```python
from build123d import *

# Parameters (mm, degrees)
SALIENTE_EXTRUIR1_DEPTH = 2.5
SALIENTE_EXTRUIR2_DEPTH = 2.5
CROQUIS3_R              = 2.25
CROQUIS3_W              = 4
CROQUIS3_H              = 100.57
CORTAR_EXTRUIR1_DEPTH   = 10
CORTAR_EXTRUIR3_DEPTH   = 82
CORTAR_EXTRUIR4_DEPTH   = 90


with BuildPart() as part:
    # Croquis1 → Saliente-Extruir1 (new body)
    with BuildSketch(Plane(origin=(0, 0, 0), x_dir=(0, 0, -1), z_dir=(1, 0, 0))):
        Polygon((-49.88, -57.285), (49.88, -57.285), (81.7, -24.565), (81.7, 25.235), (49.65, 57.285), (-49.95, 57.285), (-81.7, 24.905), (-81.7, -24.565), align=None)
    extrude(amount=SALIENTE_EXTRUIR1_DEPTH)

    # Croquis2 → Saliente-Extruir2 (add)
    with BuildSketch(Plane(origin=(2.5, 0, 0), x_dir=(0, 0, -1), z_dir=(1, 0, 0))):
        Polygon((81.7, 25.235), (49.65, 57.285), (60.256601718, 67.891601718), (92.306601718, 35.841601718), align=None)
        Polygon((-81.7, 24.905), (-49.95, 57.285), (-60.660282007, 67.786897892), (-92.410282007, 35.406897892), align=None)
        Polygon((-81.7, -24.565), (-49.88, -57.285), (-60.633463585, -67.742677606), (-92.453463585, -35.022677606), align=None)
        Polygon((49.88, -57.285), (81.7, -24.565), (92.453463585, -35.022677606), (60.633463585, -67.742677606), align=None)
    extrude(amount=-SALIENTE_EXTRUIR2_DEPTH)

    # Croquis3 → Cortar-Extruir1 (cut)
    with BuildSketch(Plane(origin=(2.5, 0, 0), x_dir=(0, 0, -1), z_dir=(1, 0, 0))):
        with Locations((-76.540373615, 33.850995118)):
            Circle(CROQUIS3_R)
        with Locations((-59.042204467, 51.550828198)):
            Circle(CROQUIS3_R)
        with Locations((76.301473252, 34.051102275)):
            Circle(CROQUIS3_R)
        with Locations((58.757017396, 51.705056035)):
            Circle(CROQUIS3_R)
        with Locations((76.369576687, -33.391936282)):
            Circle(CROQUIS3_R)
        with Locations((58.860810215, -51.081286502)):
            Circle(CROQUIS3_R)
        with Locations((-58.938482889, -51.164964143)):
            Circle(CROQUIS3_R)
        with Locations((-76.472362613, -33.500506143)):
            Circle(CROQUIS3_R)
        with BuildLine():
            Line((-8.35, 0), (-8.35, -10.698407243))
            Line((-8.35, -10.698407243), (8.347094832, -10.698407243))
            Line((8.347094832, -10.698407243), (8.321717757, -0.686668462))
            ThreePointArc((8.321717757, -0.686668462), (0.343625327, 8.342926443), (-8.35, 0))
        make_face()
        Polygon((23.469483411, 50.346823407), (23.732824148, -50.222831816), (27.732810435, -50.212357888), (27.469469698, 50.357297335), align=None)
        with Locations((-41.664502762, 0)):
            Rectangle(CROQUIS3_W, CROQUIS3_H)
        with Locations((-25.751234947, 0)):
            Rectangle(CROQUIS3_W, CROQUIS3_H)
        Polygon((39.382696671, 50.388492013), (39.646037409, -50.18116321), (43.646023696, -50.170689282), (43.382682959, 50.398965941), align=None)
    extrude(amount=-CORTAR_EXTRUIR1_DEPTH, mode=Mode.SUBTRACT)

    # Croquis4 → Cortar-Extruir3 (cut)
    with BuildSketch(Plane(origin=(0, -28.144978127, 27.597376638), x_dir=(1, 0, 0), z_dir=(0, -0.7140188004824893, 0.7001265261062083))):
        Polygon((0, 90.771987132), (2.5, 90.771987132), (2.5, 85.771987132), align=None)
        Polygon((2.5, -90.72187848), (0, -90.72187848), (2.5, -85.72187848), align=None)
    extrude(amount=-CORTAR_EXTRUIR3_DEPTH, mode=Mode.SUBTRACT)

    # Croquis6 → Cortar-Extruir4 (cut)
    with BuildSketch(Plane(origin=(0, -28.2325, -28.2325), x_dir=(1, 0, 0), z_dir=(0, -0.7071067811865475, -0.7071067811865477))):
        Polygon((0, -90.614463646), (2.5, -85.614463646), (2.5, -90.614463646), align=None)
        Polygon((0, 90.775639979), (2.5, 90.775639979), (2.5, 85.775639979), align=None)
    extrude(amount=-CORTAR_EXTRUIR4_DEPTH, mode=Mode.SUBTRACT)


solid = part.part
```
Verification items for the finished model (mm, model axes). A direction names the side the tool comes from. Round coordinates to 2 decimals unless told otherwise and drop trailing zeros. Write each loop counter-clockwise with the first axis right and the second up, starting at its lowest first coordinate (ties: lowest second). Pieces come first, ordered by that corner, then holes.
1. Draft check along Z on faces 4 (the flat face through (1.27, 29.06, 85.94)), 5 (the cylindrical face through (1.268, -35.497, 75.434)), 6 (the flat face through (1.23, -49.96, -74.62)), 7 (the cylindrical face through (1.268, 50.182, 60.828)). Enter one of: +Z half, -Z half, draft (parallel to the pull), parting line (faces both ways), or undercut.
2. Scan lines: L1, parallel to Y at x = 1.7, z = 43 (3 decimals); L2, parallel to Z at x = 2.3, y = -15.5; L3, parallel to Z at x = 0.45, y = 4. Record each from-to range of solid material in increasing order.
3. Access from +Z, -Z, +X, -X, +Y, -Y to the whole of each face (thin tool, end or side, straight path). Record for faces 1 (the cylindrical face through (1.268, 8.333, -0.532)), 2 (the flat face through (1.27, -28.56, -85.81)), 3 (the flat face through (1.267, 61.296, 54.04)).
4. Gauge pin test, flat ends, axial feed: P1, Ø0.8, axis at x = 1.5, y = -7, coming from the -Z side; P2, Ø1, axis at x = 1, z = -9, coming from the -Y side (3 decimals); P3, Ø1.2, axis at x = 1.5, y = -12, coming from the +Z side. Record the tip position at first contact, or that the pin passes through.
5. Section check B-B on z = -21. Enter the section's corners in (x, y) (3 decimals).
6. Section check A-A on z = 0. Enter the section's corners in (x, y) (3 decimals).
7. Section check C-C on x = 1.2. State how many separate pieces and enclosed holes the cut face has, plus the area to 3 significant figures.
Answer:
1. face 4: +Z half
1. face 5: undercut
1. face 6: -Z half
1. face 7: undercut
2. L1: y = -57.285 to -50.285, 50.285 to 57.285
2. L2: z = -81.7 to -43.56, -39.56 to -27.64, -23.64 to 23.75, 27.75 to 39.66, 43.66 to 81.7
2. L3: z = -81.7 to -43.5, -39.5 to -27.59, -23.59 to -7.33, 7.33 to 23.75, 27.75 to 39.66, 43.66 to 81.7
3. face 1: +X, -X
3. face 2: -Z, +X, -X
3. face 3: +X, -X, +Y
4. P1: stops at z = -81.7
4. P2: stops at y = -57.285
4. P3: stops at z = 81.7
5. outline: (0, -57.285) - (2.5, -57.285) - (2.5, 57.285) - (0, 57.285) - close
6. outline: (0, -57.285) - (2.5, -57.285) - (2.5, -10.698) - (0, -10.698) - close; (0, 8.35) - (2.5, 8.35) - (2.5, 57.285) - (0, 57.285) - close
7. separate pieces: 1
7. enclosed holes: 13
7. area: 16,900 mm2
